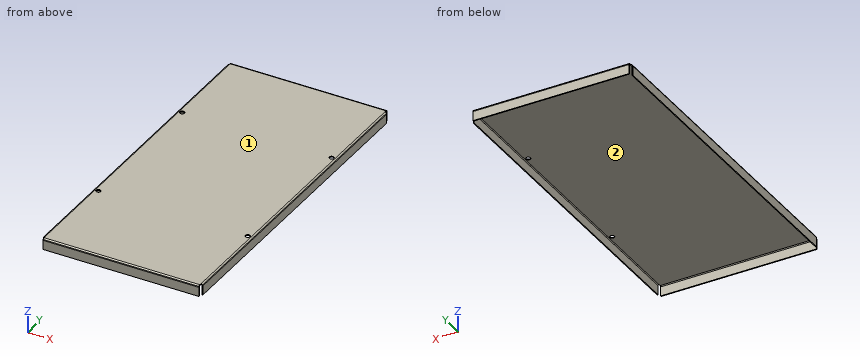
```python
from build123d import *

# Parameters (mm, degrees)
CROQUIS1_W                   = 274.574
CROQUIS1_H                   = 569.976
BRIDA_BASE1_DEPTH            = 1.524
CROQUIS6_W                   = 3.1242
CROQUIS6_H                   = 6.35
CORTAR_EXTRUIR1_DEPTH        = 317.335586188
BRIDA_START                  = -134.1628
BRIDA_DE_ARISTA1_DEPTH       = 268.3256
BRIDA_START_2                = 6.35
BRIDA_DE_ARISTA1_2_DEPTH     = 557.276
BRIDA_DE_ARISTA1_3_DEPTH     = 268.3256
BRIDA_DE_ARISTA1_4_OUTLINE_W = 0.1524
BRIDA_DE_ARISTA1_4_OUTLINE_H = 1.524
BRIDA_DE_ARISTA1_4_DEPTH     = 0.0762
BRIDA_START_3                = 134.0866
BRIDA_DE_ARISTA1_5_OUTLINE_W = 0.1524
BRIDA_DE_ARISTA1_5_OUTLINE_H = 1.524
BRIDA_DE_ARISTA1_5_DEPTH     = 0.0762
BRIDA_DE_ARISTA1_6_DEPTH     = 557.276
CROQUIS19_R                  = 3.9624
CORTAR_EXTRUIR2_DEPTH        = 317.905006292


# Read off the part's stored shape, not the designer's step: Brida de arista1
# Sheet-metal steps are written as plain solids
with BuildPart() as part:
    # Croquis1 → Brida base1 (new body)
    with BuildSketch(Plane.XY):
        Rectangle(CROQUIS1_W, CROQUIS1_H)
    extrude(amount=-BRIDA_BASE1_DEPTH)

    # Croquis6 → Cortar-Extruir1 (cut, through all)
    with BuildSketch(Plane.XY):
        with Locations((135.7249, 281.813)):
            Rectangle(CROQUIS6_W, CROQUIS6_H)
        with Locations((-135.7249, 281.813)):
            Rectangle(CROQUIS6_W, CROQUIS6_H)
        with Locations((-135.7249, -281.813)):
            Rectangle(CROQUIS6_W, CROQUIS6_H)
        with Locations((135.7249, -281.813)):
            Rectangle(CROQUIS6_W, CROQUIS6_H)
    extrude(amount=-CORTAR_EXTRUIR1_DEPTH, mode=Mode.SUBTRACT)

    # Brida de arista1 outline → Brida de arista1 (add)
    with BuildSketch(Plane.YZ.offset(BRIDA_START)):
        with BuildLine():
            Line((284.988, -19.05), (284.988, -3.048))
            ThreePointArc((284.988, -3.048), (284.884141918, -2.259119551), (284.579645431, -1.524))
            Line((284.579645431, -1.524), (281.94, -1.524))
            ThreePointArc((281.94, -1.524), (283.017630735, -1.970369265), (283.464, -3.048))
            Line((283.464, -3.048), (283.464, -19.05))
            Line((283.464, -19.05), (284.988, -19.05))
        make_face()
        with BuildLine():
            ThreePointArc((-283.464, -3.048), (-283.017630735, -1.970369265), (-281.94, -1.524))
            Line((-281.94, -1.524), (-284.579645431, -1.524))
            ThreePointArc((-284.579645431, -1.524), (-284.884141918, -2.259119551), (-284.988, -3.048))
            Line((-284.988, -3.048), (-284.988, -19.05))
            Line((-284.988, -19.05), (-283.464, -19.05))
            Line((-283.464, -19.05), (-283.464, -3.048))
        make_face()
    extrude(amount=BRIDA_DE_ARISTA1_DEPTH)

    # Brida de arista1 2 outline → Brida de arista1 2 (add)
    with BuildSketch(Plane(origin=(0, 284.988, -1.524), x_dir=(-1, 0, 0), z_dir=(0, -1, 0)).offset(BRIDA_START_2)):
        with BuildLine():
            Line((-135.763, 1.524), (-135.763, 17.526))
            Line((-135.763, 17.526), (-137.287, 17.526))
            Line((-137.287, 17.526), (-137.287, 1.524))
            ThreePointArc((-137.287, 1.524), (-137.183141918, 0.735119551), (-136.878645431, 0))
            Line((-136.878645431, 0), (-134.239, 0))
            ThreePointArc((-134.239, 0), (-135.316630735, 0.446369265), (-135.763, 1.524))
        make_face()
        with BuildLine():
            ThreePointArc((135.763, 1.524), (135.316630735, 0.446369265), (134.239, 0))
            Line((134.239, 0), (136.878645431, 0))
            ThreePointArc((136.878645431, 0), (137.183141918, 0.735119551), (137.287, 1.524))
            Line((137.287, 1.524), (137.287, 17.526))
            Line((137.287, 17.526), (135.763, 17.526))
            Line((135.763, 17.526), (135.763, 1.524))
        make_face()
    extrude(amount=BRIDA_DE_ARISTA1_2_DEPTH)

    # Brida de arista1 3 outline → Brida de arista1 3 (cut)
    with BuildSketch(Plane.YZ.offset(BRIDA_START)):
        with BuildLine():
            ThreePointArc((281.94, 0), (283.464, -0.408354569), (284.579645431, -1.524))
            Line((284.579645431, -1.524), (284.988, -1.524))
            Line((284.988, -1.524), (284.988, 0))
            Line((284.988, 0), (281.94, 0))
        make_face()
        with BuildLine():
            ThreePointArc((-284.579645431, -1.524), (-283.464, -0.408354569), (-281.94, 0))
            Line((-281.94, 0), (-284.988, 0))
            Line((-284.988, 0), (-284.988, -1.524))
            Line((-284.988, -1.524), (-284.579645431, -1.524))
        make_face()
    extrude(amount=BRIDA_DE_ARISTA1_3_DEPTH, mode=Mode.SUBTRACT)

    # Brida de arista1 4 outline → Brida de arista1 4 (cut)
    with BuildSketch(Plane.YZ.offset(BRIDA_START)):
        with Locations((278.7142, -0.762)):
            Rectangle(BRIDA_DE_ARISTA1_4_OUTLINE_W, BRIDA_DE_ARISTA1_4_OUTLINE_H)
        with Locations((-278.7142, -0.762)):
            Rectangle(BRIDA_DE_ARISTA1_4_OUTLINE_W, BRIDA_DE_ARISTA1_4_OUTLINE_H)
    extrude(amount=BRIDA_DE_ARISTA1_4_DEPTH, mode=Mode.SUBTRACT)

    # Brida de arista1 5 outline → Brida de arista1 5 (cut)
    with BuildSketch(Plane.YZ.offset(BRIDA_START_3)):
        with Locations((278.7142, -0.762)):
            Rectangle(BRIDA_DE_ARISTA1_5_OUTLINE_W, BRIDA_DE_ARISTA1_5_OUTLINE_H)
        with Locations((-278.7142, -0.762)):
            Rectangle(BRIDA_DE_ARISTA1_5_OUTLINE_W, BRIDA_DE_ARISTA1_5_OUTLINE_H)
    extrude(amount=BRIDA_DE_ARISTA1_5_DEPTH, mode=Mode.SUBTRACT)

    # Brida de arista1 6 outline → Brida de arista1 6 (cut)
    with BuildSketch(Plane(origin=(0, 284.988, -1.524), x_dir=(-1, 0, 0), z_dir=(0, -1, 0)).offset(BRIDA_START_2)):
        with BuildLine():
            ThreePointArc((-134.239, -1.524), (-135.763, -1.115645431), (-136.878645431, 0))
            Line((-136.878645431, 0), (-137.287, 0))
            Line((-137.287, 0), (-137.287, -1.524))
            Line((-137.287, -1.524), (-134.239, -1.524))
        make_face()
        with BuildLine():
            Line((137.287, 0), (136.878645431, 0))
            ThreePointArc((136.878645431, 0), (135.763, -1.115645431), (134.239, -1.524))
            Line((134.239, -1.524), (137.287, -1.524))
            Line((137.287, -1.524), (137.287, 0))
        make_face()
    extrude(amount=BRIDA_DE_ARISTA1_6_DEPTH, mode=Mode.SUBTRACT)

    # Croquis19 → Cortar-Extruir2 (cut, through all)
    with BuildSketch(Plane.XY):
        with Locations((-128.651, 127)):
            Circle(CROQUIS19_R)
        with Locations((-128.651, -127)):
            Circle(CROQUIS19_R)
        with Locations((128.651, 127)):
            Circle(CROQUIS19_R)
        with Locations((128.651, -127)):
            Circle(CROQUIS19_R)
    extrude(amount=-CORTAR_EXTRUIR2_DEPTH, mode=Mode.SUBTRACT)


solid = part.part
```
Build history of the part. All positions in model axes, mm. Face numbers are marked on the shaded views. Coordinates: 2 decimals unless noted, no trailing zeros. Write each loop counter-clockwise with the first axis right and the second up, starting at its lowest first coordinate (ties: lowest second). Pieces come first, ordered by that corner, then holes.
1. Pull direction Y, two halves, no side cores. Call the marked faces 1 and 2: released by +Y, released by -Y, zero draft, split by the parting line, or undercut.
Answer block:
face 1: zero draft
face 2: undercut
2. Band-saw the part on A-A, the plane z = -14.25. Give the cut face in (x, y), and give its area (3 significant figures).
Answer block:
outline: (-137.29, -278.64) - (-135.76, -278.64) - (-135.76, 278.64) - (-137.29, 278.64) - close; (-134.16, -284.99) - (134.16, -284.99) - (134.16, -283.46) - (-134.16, -283.46) - close; (-134.16, 283.46) - (134.16, 283.46) - (134.16, 284.99) - (-134.16, 284.99) - close; (135.76, -278.64) - (137.29, -278.64) - (137.29, 278.64) - (135.76, 278.64) - close
area: 2,520 mm2
3. Band-saw the part on C-C, the plane x = -62.5. Give the cut face in (y, z).
Answer block:
outline: (-284.99, -19.05) - (-283.46, -19.05) - (-283.46, -3.05) arc R1.52 cw to (-281.94, -1.52) - (281.94, -1.52) arc R1.52 cw to (283.46, -3.05) - (283.46, -19.05) - (284.99, -19.05) - (284.99, -3.05) arc R3.05 ccw to (281.94, 0) - (-281.94, 0) arc R3.05 ccw to (-284.99, -3.05) - close
4. Drill centre lines: probe 1 along Y at (x, z) = (-94.5, -7.5); probe 2 along X at (y, z) = (32.5, -14); probe 3 along Z at (x, y) = (20.5, -24.5). Where is each one in solid material? Low to high.
Answer block:
probe 1: y = -284.99 to -283.46, 283.46 to 284.99
probe 2: x = -137.29 to -135.76, 135.76 to 137.29
probe 3: z = -1.52 to 0
5. Band-saw the part on B-B, the plane y = 52.5. Give the cut face in (x, z), and give its area (3 significant figures).
Answer block:
outline: (-137.29, -19.05) - (-135.76, -19.05) - (-135.76, -3.05) arc R1.52 cw to (-134.24, -1.52) - (134.24, -1.52) arc R1.52 cw to (135.76, -3.05) - (135.76, -19.05) - (137.29, -19.05) - (137.29, -3.05) arc R3.05 ccw to (134.24, 0) - (-134.24, 0) arc R3.05 ccw to (-137.29, -3.05) - close
area: 469 mm2
6. Drop flat-ended pins along their axis: pin 1 (1.6 mm diameter, centred on x = 136, z = -5, fed in from +Y); pin 2 (10 mm diameter, centred on x = -55.5, y = 100.5, fed in from -Z); pin 3 (1 mm diameter, centred on x = -136.5, z = -14, fed in from -Y). Give the stop position or say it passes through.
Answer block:
pin 1: stops at y = 278.64
pin 2: stops at z = -1.52
pin 3: stops at y = -278.64
